The drawing under review shows one solid part. Ordinate dimensions are in mm from its lowest x, y, z. A direction names the side the tool comes from. Coordinates: 2 decimals unless noted, no trailing zeros. Loops run counter-clockwise (first coordinate to the right, second up) from the corner with the lowest first, then second, coordinate; pieces in that order, holes last. Notation, with made-up numbers: M -33,37 L -20,37 A17 ccw -20,50 Z; hole C 48,8.25 d5. An arc over 180 degrees is marked long. Put each result on its own line as item: value.
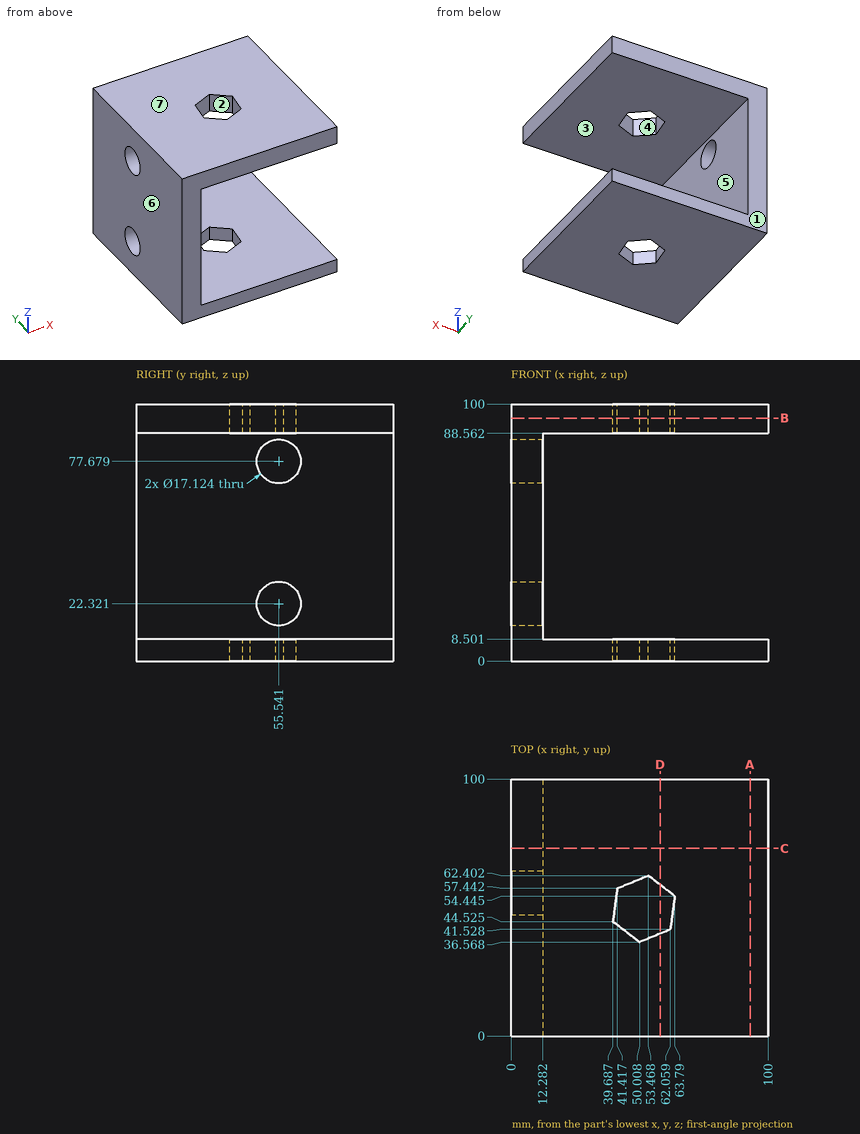
(1) Add section B-B (z = 94.5). Write out the cut boundary in (x, y) (1 decimal), plus the area to 3 significant figures.
Determined:
outline: M 0,0 L 100,0 L 100,100 L 0,100 Z; hole M 39.7,44.5 L 50,36.6 L 62.1,41.5 L 63.8,54.4 L 53.5,62.4 L 41.4,57.4 Z
area: 9,560 mm^2
(2) Wall thickness on line 1 along Z through (x, y) = (96.5, 47); line 2 along X through (y, z) = (60.5, 54); line 3 along X through (y, z) = (61.5, 8) (1 decimal): over which ranges is each line inside the solid? List them lowest first. Write a range as [from, to].
Determined:
line 1: z = [0, 8.5], [88.56, 100]
line 2: x = [0, 12.28]
line 3: x = [0, 51.3], [54.6, 100]
(3) For pin 1 (1 mm diameter, centred on y = 31.5, z = 35, fed in from +X), flat-tipped, find the tip position at first contact; note if it passes through.
Determined:
pin 1: stops at x = 12.28
(4) Draft analysis for pull direction X (two halves, no side actions). For the marked faces 4, 5, 6 and 7, state which applies: +X half, -X half, draft (parallel to the pull), parting line (faces both ways), or undercut.
Determined:
face 4: undercut
face 5: +X half
face 6: -X half
face 7: draft
(5) Add section D-D (x = 58). Write out the cut boundary in (y, z), plus the area to 3 significant figures.
Determined:
outline: M 0,0 L 39.86,0 L 39.86,8.5 L 0,8.5 Z; M 0,88.56 L 39.86,88.56 L 39.86,100 L 0,100 Z; M 58.91,0 L 100,0 L 100,8.5 L 58.91,8.5 Z; M 58.91,88.56 L 100,88.56 L 100,100 L 58.91,100 Z
area: 1,610 mm^2
(6) Add section C-C (y = 73). Write out the cut boundary in (x, z), plus the area to 3 significant figures.
Determined:
outline: M 0,0 L 100,0 L 100,8.5 L 12.28,8.5 L 12.28,88.56 L 100,88.56 L 100,100 L 0,100 Z
area: 2,980 mm^2
(7) Tool access review of the marked faces 1, 2 and 3: name each direction out of +Z, -Z, +X, -X, +Y, -Y from which nothing blocks a thin tool from reaching the whole face with its end or side.
Determined:
face 1: +Z, -Z, +X, -X, +Y
face 2: +Z, -Z
face 3: +X, +Y, -Y
(8) Add section A-A (x = 93). Write out the cut boundary in (y, z).
Determined:
outline: M 0,0 L 100,0 L 100,8.5 L 0,8.5 Z; M 0,88.56 L 100,88.56 L 100,100 L 0,100 Z
